Geometry: final body of the model. Coordinates: model frame, mm. Face numbers are marked on the shaded views. Coordinates: 2 decimals unless noted, no trailing zeros. Loops run counter-clockwise (first coordinate to the right, second up) from the corner with the lowest first, then second, coordinate; pieces in that order, holes last. Notation, with made-up numbers: (1, -38.5) - (32, -38.5) arc R5 ccw to (32, -34.5) - close; hole circle Ø5 at (89, -12.5). An arc over 180 degrees is marked (long way). Answer in a Markdown table with one row per item.
from build123d import *

# Parameters (mm, degrees)
SKETCH1_R           = 2.71553392
SKETCH1_R_2         = 3.710832544
SKETCH1_W           = 12.7
SKETCH1_H           = 3.175
BOSS_EXTRUDE1_DEPTH = 3.175


with BuildPart() as part:
    # Sketch1 → Boss-Extrude1 (new body)
    with BuildSketch(Plane.XY):
        with BuildLine():
            Line((-19.05, -124.386703653), (-19.05, -93.3255592))
            ThreePointArc((-19.05, -93.3255592), (-52.146864666, -79.707383632), (-77.881676461, -54.836183051))
            Line((-77.881676461, -54.836183051), (-93.458011754, -65.803419661))
            ThreePointArc((-93.458011754, -65.803419661), (-77.110154229, -84.371287265), (-57.15, -98.986703653))
            Line((-57.15, -98.986703653), (-57.15, -124.386703653))
            Line((-57.15, -124.386703653), (-19.05, -124.386703653))
        make_face()
        with Locations((-76.904233533, -75.837226531)):
            Circle(SKETCH1_R, mode=Mode.SUBTRACT)
        with Locations((-62.697046078, -83.364915406)):
            Circle(SKETCH1_R_2, mode=Mode.SUBTRACT)
        with Locations((-38.1, -103.749203653)):
            Rectangle(SKETCH1_W, SKETCH1_H, mode=Mode.SUBTRACT)
    extrude(amount=BOSS_EXTRUDE1_DEPTH)


solid = part.part
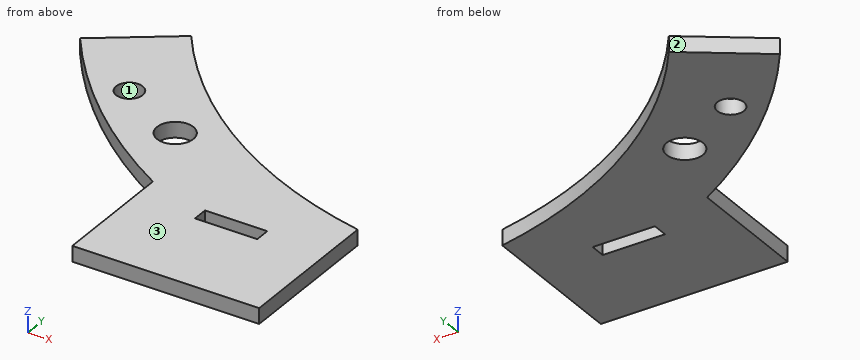
(1) Cut plane D-D on x = -83.5. Output: boundary loops of the cut face in (y, z) (3 decimals), then the cut area to 3 significant figures.
Verdict:
| item | result |
|---|---|
| outline | (-78.053, 0) - (-58.792, 0) - (-58.792, 3.175) - (-78.053, 3.175) - close |
| area | 61.2 mm² |
(2) Pull-direction query (X, two-part tool) for the marked faces 1, 2 and 3; classes: pulls with the +X half, pulls with the -X half, needs draft (parallel to the pull), parting line crosses it, or undercut.
Verdict:
| item | result |
|---|---|
| face 1 | undercut |
| face 2 | pulls with the -X half |
| face 3 | needs draft |
(3) First-contact query: pin 1 Ø1 at (x, z) = (-74, 2) entering from +Y; pin 2 Ø1 at (y, z) = (-103.5, 1) entering from -X. Flat tips, straight axial feed; report the tip coordinate or a pass-through.
Verdict:
| item | result |
|---|---|
| pin 1 | stops at y = -59.35 |
| pin 2 | stops at x = -57.15 |
(4) Cut plane C-C on y = -111. Output: boundary loops of the cut face in (x, z) (3 decimals), then the cut area to 3 significant figures.
Verdict:
| item | result |
|---|---|
| outline | (-57.15, 0) - (-19.05, 0) - (-19.05, 3.175) - (-57.15, 3.175) - close |
| area | 121 mm² |
(5) Cut plane A-A on y = -75. Output: boundary loops of the cut face in (x, z) (3 decimals), then the cut area to 3 significant figures.
Verdict:
| item | result |
|---|---|
| outline | (-86.252, 0) - (-79.487, 0) - (-79.487, 3.175) - (-86.252, 3.175) - close; (-74.321, 0) - (-58.716, 0) - (-58.716, 3.175) - (-74.321, 3.175) - close |
| area | 71.0 mm² |
(6) Ray query, probe 1 along X at (y, z) = (-105, 0.2); probe 2 along Y at (x, z) = (-66, 2.4); probe 3 along X at (y, z) = (-113, 0.8). Return the intervals inside material, ascending.
Verdict:
| item | result |
|---|---|
| probe 1 | x = -57.15 to -44.45, -31.75 to -19.05 |
| probe 2 | y = -93.32 to -85.06, -81.67 to -68.68 |
| probe 3 | x = -57.15 to -19.05 |
(7) Cut plane B-B on z = 0.55. Output: boundary loops of the cut face in (x, y), then the cut area to 3 significant figures.
Verdict:
| item | result |
|---|---|
| outline | (-93.46, -65.8) arc R114.3 ccw to (-57.15, -98.99) - (-57.15, -124.39) - (-19.05, -124.39) - (-19.05, -93.33) arc R95.25 cw to (-77.88, -54.84) - close; hole circle Ø5.43 at (-76.9, -75.84); hole circle Ø7.42 at (-62.7, -83.36); hole (-44.45, -105.34) - (-31.75, -105.34) - (-31.75, -102.16) - (-44.45, -102.16) - close |
| area | 2,100 mm² |
